```python
from build123d import *

# Parameters (mm, degrees)
SKETCH1_W           = 500
SKETCH1_H           = 200
SKETCH1_R           = 2.75
BOSS_EXTRUDE1_DEPTH = 3.175
SKETCH2_W           = 500
SKETCH2_H           = 200
SKETCH2_W_2         = 499
SKETCH2_H_2         = 199
CUT_EXTRUDE1_DEPTH  = 3.175
BOSS_EXTRUDE2_DEPTH = 3.175
FILLET1_R           = 1


with BuildPart() as part:
    # Sketch1 → Boss-Extrude1 (new body)
    with BuildSketch(Plane.YZ):
        Rectangle(SKETCH1_W, SKETCH1_H)
        with Locations(Location((237.5, 84, 0), (0, 0, 270))):
            Circle(SKETCH1_R, mode=Mode.SUBTRACT)
        with Locations(Location((-237.5, 84, 0), (0, 0, 270))):
            Circle(SKETCH1_R, mode=Mode.SUBTRACT)
        with Locations(Location((237.5, -84, 0), (0, 0, 270))):
            Circle(SKETCH1_R, mode=Mode.SUBTRACT)
        with Locations(Location((-237.5, -84, 0), (0, 0, 270))):
            Circle(SKETCH1_R, mode=Mode.SUBTRACT)
    extrude(amount=BOSS_EXTRUDE1_DEPTH)

    # Sketch2 → Cut-Extrude1 (cut)
    with BuildSketch(Plane.YZ.offset(3.175)):
        Rectangle(SKETCH2_W, SKETCH2_H)
        Rectangle(SKETCH2_W_2, SKETCH2_H_2, mode=Mode.SUBTRACT)
    extrude(amount=-CUT_EXTRUDE1_DEPTH, mode=Mode.SUBTRACT)

    # Sketch3 → Boss-Extrude2 (add, through all)
    with BuildSketch(Plane.YZ.offset(3.175)):
        Polygon((222, -99.5), (-222, -99.5), (-222, -151.5), (-193.6, -151.5), (-193.6, -131.5), (-150.9, -131.5), (-150.9, -151.5), (-78.77, -151.5), (-78.77, -131.5), (-36.07, -131.5), (-36.07, -151.5), (36.07, -151.5), (36.07, -131.5), (78.77, -131.5), (78.77, -151.5), (150.9, -151.5), (150.9, -131.5), (193.6, -131.5), (193.6, -151.5), (222, -151.5), align=None)
    extrude(amount=-BOSS_EXTRUDE2_DEPTH)

    # Fillet1
    fillet1_edges = [part.edges().sort_by_distance(p)[0] for p in [
        (1.5875, 193.6, -151.5),
        (1.5875, 193.6, -131.5),
        (1.5875, 150.9, -131.5),
        (1.5875, 150.9, -151.5),
        (1.5875, 78.77, -151.5),
        (1.5875, 78.77, -131.5),
        (1.5875, 36.07, -131.5),
        (1.5875, 36.07, -151.5),
        (1.5875, -36.07, -151.5),
        (1.5875, -36.07, -131.5),
        (1.5875, -78.77, -131.5),
        (1.5875, -78.77, -151.5),
        (1.5875, -150.9, -151.5),
        (1.5875, -150.9, -131.5),
        (1.5875, -193.6, -131.5),
        (1.5875, -193.6, -151.5),
    ]]
    fillet(fillet1_edges, radius=FILLET1_R)


solid = part.part
```
Check sheet for the modelled part. Datum: model origin and axes. Units: mm. Coordinates: 2 decimals unless noted, no trailing zeros. Order: outer loops, then holes, each group sorted by start corner. A loop starts at its lowest first (then second) coordinate and runs counter-clockwise, first axis right, second up. Notation, with made-up numbers: M -10,46.25 L 2,46.25 A21 cw 2,61.25 Z; hole C -14.75,69 d5. An arc over 180 degrees is marked long. Write each question's results on one line, items separated by ' | '. Start each with the question number.
1. Cross-section at A-A on x = 1.45. State how many separate pieces and enclosed holes the cut face has, and give its area (3 significant figures).
2. Material ranges on probe 1 along Z at (x, y) = (1.9, 237.5); probe 2 along Y at (x, z) = (1.25, 84); probe 3 along Y at (x, z) = (0.1, -117.5), recorded low to high.
3. Go/stop test with flat-tipped pins: P1, Ø4.5, axis at y = 237.5, z = 84, coming from the +X side; P2, Ø1.6, axis at x = 2, z = -143, coming from the -Y side; P3, Ø1.6, axis at x = 1, y = 167.5, coming from the -Z side; P4, Ø1.6, axis at x = 2, z = -118.5, coming from the +Y side. Record where each tip stops, or that it passes through.
4. Cross-section at B-B on y = -175. Record the cut outline in (x, z) (3 decimals).
Checks:
1) separate pieces: 1 | enclosed holes: 4 | area: 119,000 mm²
2) probe 1: z = -99.5 to -86.75, -81.25 to 81.25, 86.75 to 99.5 | probe 2: y = -249.5 to -240.25, -234.75 to 234.75, 240.25 to 249.5 | probe 3: y = -222 to 222
3) P1: passes through | P2: stops at y = -222 | P3: stops at z = -131.5 | P4: stops at y = 222
4) outline: M 0,-131.5 L 3.175,-131.5 L 3.175,99.5 L 0,99.5 Z
